Source: CAD feature listing. Evaluate the final solid. Frame: model axes, mm. A direction names the side the tool comes from. Coordinates: 2 decimals unless noted, no trailing zeros. Loops run counter-clockwise (first coordinate to the right, second up) from the corner with the lowest first, then second, coordinate; pieces in that order, holes last.
Item 1: Section query A-A, the plane x = 0. Return the cut outline in (y, z) (3 decimals), then the cut area to 3 significant figures.
Item 2: Line query: probe 1 along X at (y, z) = (11.25, 3.4); probe 2 along Y at (x, z) = (-2.5, 3.55); probe 3 along Y at (x, z) = (-1.5, 3.05). Output: solid intervals per line, ascending.
Item 3: Section query C-C, the plane y = 12. Return the cut outline in (x, z).
Item 4: Pin query (flat end, axial travel): pin 1 Ø1 at (y, z) = (10.5, 1) entering from -X; pin 2 Ø1 at (y, z) = (0, 1.5) entering from -X; pin 3 Ø1.1 at (x, z) = (1, 2.5) entering from +Y. Return the tip coordinate at first contact, or that it passes through.
Item 5: Pull-direction query (Y, two-part tool) for faces 3 (the flat face through (5.53, 9.48, 1.8)), 4 (the cylindrical face through (-1.79, 14.41, 1.8)), 5 (the flat face through (-5, 2, 0)); classes: +Y half, -Y half, draft (parallel to the pull), parting line (faces both ways), or undercut.
Item 6: Reachability of faces 1 (the flat face through (0, 12.7, 2)), 2 (the flat face through (-5, 2, 3.658)) from +Z, -Z, +X, -X, +Y, -Y: full face, straight path, thin tool, end or side. Return the list, or none.
Item 7: Section query B-B, the plane z = 0.8. Return the cut outline in (x, y) (3 decimals), then the cut area to 3 significant figures.
Autodesk Inventor part; units mm, degrees
ref_plane "YZ Plane" through (0, 0, 0) normal (1, 0, 0) x (0, 1, 0)
ref_plane "XZ Plane" through (0, 0, 0) normal (0, 1, 0) x (-1, 0, 0)
ref_plane "XY Plane" through (0, 0, 0) normal (0, 0, 1) x (1, 0, 0)
sketch "Sketch2" plane through (0, 0, 0) normal (0, 0, 1) x (1, 0, 0)
  line L0 (0, 12.7) -> (3.6703, 12.7)
  line L1 (0, 12.7) -> (-3.6703, 12.7)
  line L2 (0, 0) -> (3.6703, 0)
  line L3 (0, 0) -> (-3.6703, 0)
  line L4 (-3.6703, 0) -> (-7.3406, 6.35)
  line L5 (-7.3406, 6.35) -> (-3.6703, 12.7)
  line L6 (3.6703, 12.7) -> (7.3406, 6.35)
  line L7 (7.3406, 6.35) -> (3.6703, 0)
  line L8 (0, 0) -> (0, 6.35)
  circle A0 centre (0, 6.35) radius 8.255
  dimension "d11" = 6.35
  dimension "d12" = 16.51
extrude "Extrusion2" add sketch "Sketch2" along normal blind 6.223
sketch "Sketch3" plane through (0, 6.35, 6.223) normal (0, 0, 1) x (1, 0, 0)
  line L0 (-3.6703, -6.35) -> (-7.3406, 0)
  line L1 (-7.3406, 0) -> (-3.6703, 6.35)
  line L2 (-3.6703, 6.35) -> (3.6703, 6.35)
  line L3 (3.6703, 6.35) -> (7.3406, 0)
  line L4 (7.3406, 0) -> (3.6703, -6.35)
  line L5 (3.6703, -6.35) -> (-3.6703, -6.35)
  circle A0 centre (0, 0) radius 8.255
  point P0 (0, -6.35)
extrude "Extrusion3" add sketch "Sketch3" along normal blind 3.302
sketch "Sketch4" plane through (0, 6.35, 9.525) normal (0, 0, 1) x (1, 0, 0)
  line L0 (-7.3406, 0) -> (-3.6703, 6.35)
  line L1 (-3.6703, 6.35) -> (3.6703, 6.35)
  line L2 (3.6703, 6.35) -> (7.3406, 0)
  line L3 (7.3406, 0) -> (3.6703, -6.35)
  line L4 (3.6703, -6.35) -> (-3.6703, -6.35)
  line L5 (-3.6703, -6.35) -> (-7.3406, 0)
  circle A0 centre (0, 0) radius 8.255
  point P0 (0, -6.35)
extrude "Extrusion4" add sketch "Sketch4" along normal blind 6.5786
sketch "Sketch5" plane through (0, 6.35, 16.1036) normal (0, 0, 1) x (1, 0, 0)
  line L0 (-16.3467, 15.7745) -> (15.1254, 15.7745)
  line L1 (15.1254, 15.7745) -> (15.1254, -12.8793)
  line L2 (15.1254, -12.8793) -> (-16.3467, -12.8793)
  line L3 (-16.3467, -12.8793) -> (-16.3467, 15.7745)
  point P0 (0, -6.35)
extrude "Extrusion5" cut sketch "Sketch5" against normal blind 6.5786
sketch "Sketch8" plane through (0, 6.35, 9.525) normal (0, 0, 1) x (1, 0, 0)
  line L0 (-7.3406, 0) -> (-3.6703, -6.35)
  line L1 (-3.6703, 6.35) -> (-7.3406, 0)
  line L2 (3.6703, 6.35) -> (-3.6703, 6.35)
  line L3 (7.3406, 0) -> (3.6703, 6.35)
  line L4 (3.6703, -6.35) -> (7.3406, 0)
  line L5 (-3.6703, -6.35) -> (3.6703, -6.35)
  circle A0 centre (0, 0) radius 8.255
  point P0 (0, -6.35)
extrude "Extrusion7" add sketch "Sketch8" along normal blind 15.875
sketch "Sketch9" plane through (0, 6.35, 25.4) normal (0, 0, 1) x (1, 0, 0)
  line L0 (-7.3406, 0) -> (-3.6703, 6.35)
  line L1 (-3.6703, 6.35) -> (3.6703, 6.35)
  line L2 (3.6703, 6.35) -> (7.3406, 0)
  line L3 (7.3406, 0) -> (3.6703, -6.35)
  line L4 (3.6703, -6.35) -> (-3.6703, -6.35)
  line L5 (-3.6703, -6.35) -> (-7.3406, 0)
  circle A0 centre (0, 0) radius 8.255
  point P0 (0, -6.35)
extrude "Extrusion8" cut sketch "Sketch9" against normal blind 21.7424
properties part number ".144Spacer"
Verdict:
1. outline: (-1.905, 0) - (0, 0) - (0, 3.658) - (-1.905, 3.658) - close; (12.7, 0) - (14.605, 0) - (14.605, 3.658) - (12.7, 3.658) - close
1. area: 13.9 mm2
2. probe 1: x = -6.64 to -4.51, 4.51 to 6.64
2. probe 2: y = -1.52 to 0, 12.7 to 14.22
2. probe 3: y = -1.77 to 0, 12.7 to 14.47
3. outline: (-6.02, 0) - (-4.07, 0) - (-4.07, 3.66) - (-6.02, 3.66) - close; (4.07, 0) - (6.02, 0) - (6.02, 3.66) - (4.07, 3.66) - close
4. pin 1: stops at x = -7.4
4. pin 2: stops at x = -5.82
4. pin 3: stops at y = 14.59
5. face 3: undercut
5. face 4: parting line
5. face 5: draft
6. face 1: +Z, -Z
6. face 2: +Z, +X, -X, +Y, -Y
7. outline: circle Ø16.51 at (0, 6.35); hole (-7.341, 6.35) - (-3.67, 0) - (3.67, 0) - (7.341, 6.35) - (3.67, 12.7) - (-3.67, 12.7) - close
7. area: 74.2 mm2
